Part model, mm, in its own coordinate system. A direction names the side the tool comes from. Coordinates: 2 decimals unless noted, no trailing zeros. Write each loop counter-clockwise with the first axis right and the second up, starting at its lowest first coordinate (ties: lowest second). Pieces come first, ordered by that corner, then holes. Notation, with made-up numbers: (12, 67) - (41, 67) arc R20 ccw to (41, 80) - close; hole circle Ø7 at (64.5, 88). An arc over 180 degrees is marked (long way). Use one line per item in the form item = value. Start each with the question number.
from build123d import *

# Parameters (mm, degrees)
SKETCH1_W           = 8
SKETCH1_H           = 28
BOSS_EXTRUDE1_DEPTH = 2
FILLET1_R           = 3
SKETCH2_W           = 4
SKETCH2_H           = 2
BOSS_EXTRUDE2_DEPTH = 12
FILLET2_R           = 1
SKETCH3_R           = 2
CUT_EXTRUDE3_DEPTH  = 10


with BuildPart() as part:
    # Sketch1 → Boss-Extrude1 (new body)
    with BuildSketch(Plane.XY):
        Rectangle(SKETCH1_W, SKETCH1_H)
    extrude(amount=BOSS_EXTRUDE1_DEPTH)

    # Fillet1
    fillet1_edges = [part.edges().sort_by_distance(p)[0] for p in [
        (-4, 14, 1),
        (4, 14, 1),
        (4, -14, 1),
        (-4, -14, 1),
    ]]
    fillet(fillet1_edges, radius=FILLET1_R)

    # Sketch2 → Boss-Extrude2 (add)
    with BuildSketch(Plane(origin=(0, 0, 0), x_dir=(-1, 0, 0), z_dir=(0, 0, -1))):
        with Locations((0, 10)):
            Rectangle(SKETCH2_W, SKETCH2_H)
        with Locations((0, -10)):
            Rectangle(SKETCH2_W, SKETCH2_H)
    extrude(amount=BOSS_EXTRUDE2_DEPTH)

    # Fillet2
    fillet2_edges = [part.edges().sort_by_distance(p)[0] for p in [
        (2, 11, -6),
        (-2, 11, -6),
        (-2, -11, -6),
        (2, -11, -6),
    ]]
    fillet(fillet2_edges, radius=FILLET2_R)

    # Sketch3 → Cut-Extrude3 (cut)
    with BuildSketch(Plane(origin=(0, 0, 0), x_dir=(-1, 0, 0), z_dir=(0, 0, -1))):
        Circle(SKETCH3_R)
    extrude(amount=-CUT_EXTRUDE3_DEPTH, mode=Mode.SUBTRACT)


solid = part.part
Q1. Pin check, flat tips, straight feed: P1, Ø2, axis at x = 0, z = -6.5, coming from the -Y side; P2, Ø1, axis at x = 0, z = -8, coming from the +Y side; P3, Ø4, axis at y = -9, z = -6, coming from the +X side. Stop position of each tip, or through.
Q2. Mould opens along Y. For faces 4 (the flat face through (2, -9.5, -5.9)), 5 (the cylindrical face through (0, -2, 1)), 6 (the flat face through (0, -14, 1)) say: released by +Y, released by -Y, zero draft, split by the parting line, or undercut.
Q3. Slice it at C-C (y = 0). List the corners of the cut face in (x, z).
Q4. Slice it at B-B (z = -8). List the corners of the cut face in (x, y), plus the area to 3 significant figures.
Q5. Slice it at D-D (y = 6). List the corners of the cut face in (x, z).
Q6. Which spindle directions (+Z, -Z, +X, -X, +Y, -Y) get a long thin tool onto all of the face, cutting with end or side? Do faces 1 (the flat face through (0, -11, -6)), 2 (the flat face through (-2, 9.5, -5.9)), 3 (the flat face through (2, 9.5, -5.9)). Say none if no direction does.
Q7. Slice it at A-A (x = 0). List the corners of the cut face in (y, z).
Q8. Drill centre lines: probe 1 along Y at (x, z) = (-0.5, -7.5); probe 2 along Y at (x, z) = (0, 0.7); probe 3 along Z at (x, y) = (1.75, 8.75). Where is each one in solid material? Low to high.
Solution:
q1.P1 = -11
q1.P2 = 11
q1.P3 = 2
q2.face_4 = zero draft
q2.face_5 = undercut
q2.face_6 = released by -Y
q3.outline = (-4, 0) - (-2, 0) - (-2, 2) - (-4, 2) - close; (2, 0) - (4, 0) - (4, 2) - (2, 2) - close
q4.outline = (-2, -10) arc R1 ccw to (-1, -11) - (1, -11) arc R1 ccw to (2, -10) - (2, -9) - (-2, -9) - close; (-2, 9) - (2, 9) - (2, 10) arc R1 ccw to (1, 11) - (-1, 11) arc R1 ccw to (-2, 10) - close
q4.area = 15.1 mm2
q5.outline = (-4, 0) - (4, 0) - (4, 2) - (-4, 2) - close
q6.face_1 = -Z, +X, -X, -Y
q6.face_2 = -Z, -X, +Y, -Y
q6.face_3 = -Z, +X, +Y, -Y
q7.outline = (-14, 0) - (-11, 0) - (-11, -12) - (-9, -12) - (-9, 0) - (-2, 0) - (-2, 2) - (-14, 2) - close; (2, 0) - (9, 0) - (9, -12) - (11, -12) - (11, 0) - (14, 0) - (14, 2) - (2, 2) - close
q8.probe_1 = -11 to -9, 9 to 11
q8.probe_2 = -14 to -2, 2 to 14
q8.probe_3 = 0 to 2
